Input: part model. Units: mm. Frame: model coordinates. Face numbers are marked on the shaded views. Round coordinates to 2 decimals unless told otherwise and drop trailing zeros. Loops run counter-clockwise (first coordinate to the right, second up) from the corner with the lowest first, then second, coordinate; pieces in that order, holes last.
1) First-contact query: pin 1 (1 mm diameter, centred on x = -12.5, z = 1.5, fed in from +Y); pin 2 (3 mm diameter, centred on x = -32, y = -6.5, fed in from +Z). Flat tips, straight axial feed; report the tip coordinate or a pass-through.
2) Draft query along X for the marked faces 1 and 2. Return one class per face: pulls with the +X half, pulls with the -X half, needs draft (parallel to the pull), parting line crosses it, or undercut.
3) Section A-A, the plane z = 1.45. Return loops of the section in (x, y), and give its area (3 significant figures).
4) Section C-C, the plane y = 15.5. Return loops of the section in (x, z), and give its area (3 significant figures).
5) Section B-B, the plane x = -25. Return loops of the section in (y, z), and give its area (3 significant figures).
6) Section D-D, the plane y = 21. Return loops of the section in (x, z).
7) Ray query, line 1 along Y through (x, z) = (-20, 0.8); line 2 along X through (y, z) = (0, 1.2); line 3 along X through (y, z) = (16.5, 0.25). Return the intervals inside material, ascending.
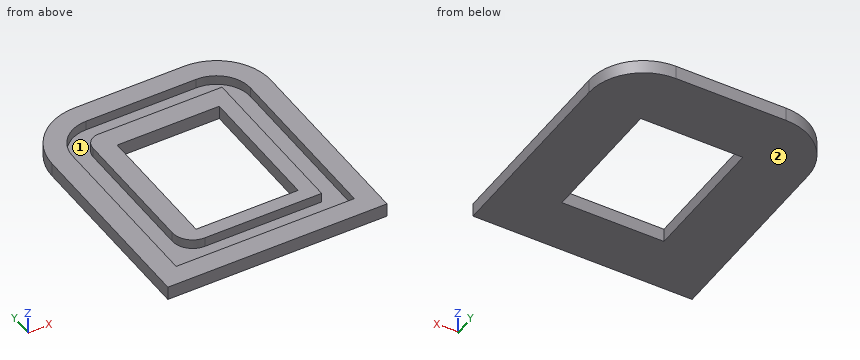
from build123d import *

# Parameters (mm, degrees)
F1_DEPTH = 0.6
F0_W     = 14.97182
F0_H     = 19.371433
F2_DEPTH = 2


with BuildPart() as f1:
    # F0 (on Top) → F1 (new body)
    with BuildSketch(Plane.XY):
        with BuildLine():
            Line((-13.600235, 22.844931), (-29.731723, 22.844931))
            ThreePointArc((-29.731723, 22.844931), (-33.267257, 21.380465), (-34.731723, 17.844931))
            Line((-34.731723, 17.844931), (-34.731723, -7.614977))
            Line((-34.731723, -7.614977), (-8.600235, -7.614977))
            Line((-8.600235, -7.614977), (-8.600235, 17.844931))
            ThreePointArc((-8.600235, 17.844931), (-10.064701, 21.380465), (-13.600235, 22.844931))
        make_face()
        with BuildLine():
            ThreePointArc((-31.731723, 17.844931), (-31.145937, 19.259145), (-29.731723, 19.844931))
            Line((-29.731723, 19.844931), (-11.600235, 19.844931))
            Line((-11.600235, 19.844931), (-11.600235, -4.614977))
            Line((-11.600235, -4.614977), (-28.731723, -4.614977))
            ThreePointArc((-28.731723, -4.614977), (-30.853044, -3.736297), (-31.731723, -1.614977))
            Line((-31.731723, -1.614977), (-31.731723, 17.844931))
        make_face(mode=Mode.SUBTRACT)
    extrude(amount=F1_DEPTH)

    # F0 (on Top) → F2 (join)
    with BuildSketch(Plane.XY):
        with BuildLine():
            Line((-13.600235, 25.844931), (-29.731723, 25.844931))
            ThreePointArc((-29.731723, 25.844931), (-35.388578, 23.501785), (-37.731723, 17.844931))
            Line((-37.731723, 17.844931), (-37.731723, -10.614977))
            Line((-37.731723, -10.614977), (-5.600235, -10.614977))
            Line((-5.600235, -10.614977), (-5.600235, 17.844931))
            ThreePointArc((-5.600235, 17.844931), (-7.943381, 23.501785), (-13.600235, 25.844931))
        make_face()
        with BuildLine():
            ThreePointArc((-34.731723, 17.844931), (-33.267257, 21.380465), (-29.731723, 22.844931))
            Line((-29.731723, 22.844931), (-13.600235, 22.844931))
            ThreePointArc((-13.600235, 22.844931), (-10.064701, 21.380465), (-8.600235, 17.844931))
            Line((-8.600235, 17.844931), (-8.600235, -7.614977))
            Line((-8.600235, -7.614977), (-34.731723, -7.614977))
            Line((-34.731723, -7.614977), (-34.731723, 17.844931))
        make_face(mode=Mode.SUBTRACT)
        with BuildLine():
            Line((-11.600235, 19.844931), (-29.731723, 19.844931))
            ThreePointArc((-29.731723, 19.844931), (-31.145937, 19.259145), (-31.731723, 17.844931))
            Line((-31.731723, 17.844931), (-31.731723, -1.614977))
            ThreePointArc((-31.731723, -1.614977), (-30.853044, -3.736297), (-28.731723, -4.614977))
            Line((-28.731723, -4.614977), (-11.600235, -4.614977))
            Line((-11.600235, -4.614977), (-11.600235, 19.844931))
        make_face()
        with Locations((-21.324334, 7.095438)):
            Rectangle(F0_W, F0_H, mode=Mode.SUBTRACT)
    extrude(amount=F2_DEPTH)


solid = f1.part
Final values:
1. pin 1: stops at y = 25.82
1. pin 2: stops at z = 2
2. face 1: undercut
2. face 2: needs draft
3. outline: (-37.73, -10.61) - (-5.6, -10.61) - (-5.6, 17.84) arc R8 ccw to (-13.6, 25.84) - (-29.73, 25.84) arc R8 ccw to (-37.73, 17.84) - close; (-31.73, -1.61) arc R3 ccw to (-28.73, -4.61) - (-11.6, -4.61) - (-11.6, 19.84) - (-29.73, 19.84) arc R2 ccw to (-31.73, 17.84) - close; hole (-34.73, -7.61) - (-8.6, -7.61) - (-8.6, 17.84) arc R5 ccw to (-13.6, 22.84) - (-29.73, 22.84) arc R5 ccw to (-34.73, 17.84) - close; hole (-28.81, -2.59) - (-13.84, -2.59) - (-13.84, 16.78) - (-28.81, 16.78) - close
3. area: 558 mm2
4. outline: (-37.73, 0) - (-28.81, 0) - (-28.81, 2) - (-31.73, 2) - (-31.73, 0.6) - (-34.73, 0.6) - (-34.73, 2) - (-37.73, 2) - close; (-13.84, 0) - (-5.6, 0) - (-5.6, 2) - (-8.6, 2) - (-8.6, 0.6) - (-11.6, 0.6) - (-11.6, 2) - (-13.84, 2) - close
4. area: 25.9 mm2
5. outline: (-10.61, 0) - (-2.59, 0) - (-2.59, 2) - (-4.61, 2) - (-4.61, 0.6) - (-7.61, 0.6) - (-7.61, 2) - (-10.61, 2) - close; (16.78, 0) - (25.84, 0) - (25.84, 2) - (22.84, 2) - (22.84, 0.6) - (19.84, 0.6) - (19.84, 2) - (16.78, 2) - close
5. area: 25.8 mm2
6. outline: (-37.08, 0) - (-6.25, 0) - (-6.25, 2) - (-9.72, 2) - (-9.72, 0.6) - (-33.61, 0.6) - (-33.61, 2) - (-37.08, 2) - close
7. line 1: y = -10.61 to -7.61, -4.61 to -2.59, 16.78 to 19.84, 22.84 to 25.84
7. line 2: x = -37.73 to -34.73, -31.73 to -28.81, -13.84 to -11.6, -8.6 to -5.6
7. line 3: x = -37.73 to -28.81, -13.84 to -5.6
